Geometry check sheet. Reference: drawing and pictorial views, mm from the part's lowest x, y, z. Coordinates: 2 decimals unless noted, no trailing zeros. Write each loop counter-clockwise with the first axis right and the second up, starting at its lowest first coordinate (ties: lowest second). Pieces come first, ordered by that corner, then holes. Notation, with made-up numbers: M -4.75,17 L 22.25,17 A33 cw 22.25,45 Z; hole C 26,36.25 d4. An arc over 180 degrees is marked long. One line per item, written item: value.
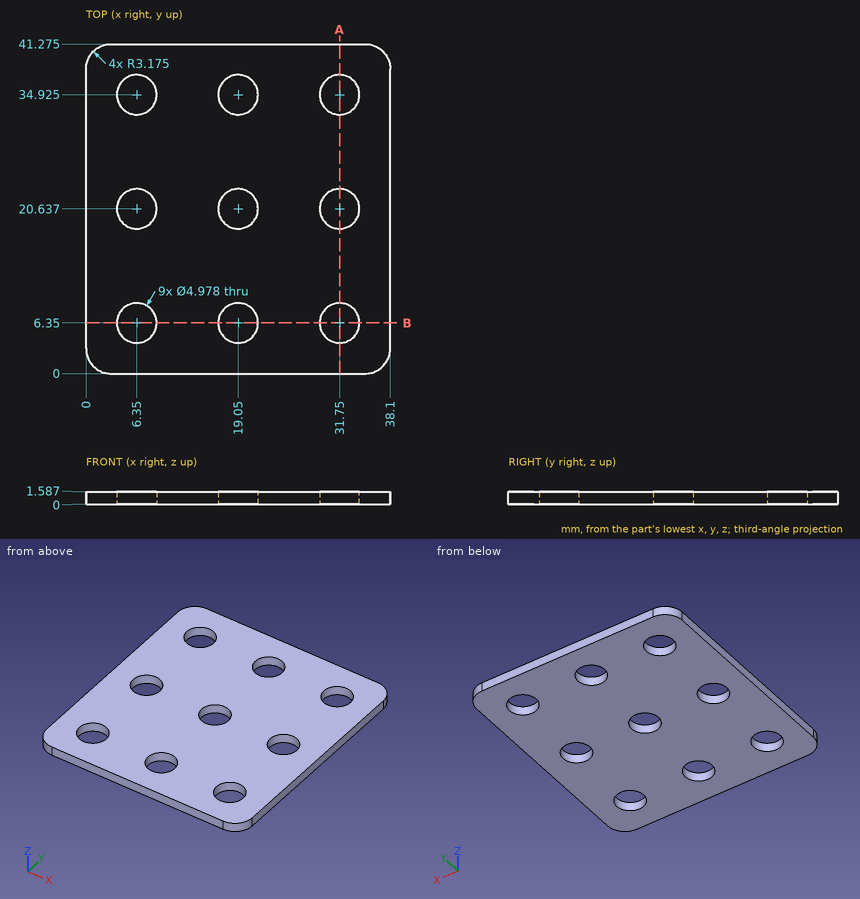
Item 1: Cross-section at A-A, the plane x = 31.75. Enter the section's corners in (y, z) (1 decimal).
The answers:
outline: M 0,0 L 3.9,0 L 3.9,1.6 L 0,1.6 Z; M 8.8,0 L 18.1,0 L 18.1,1.6 L 8.8,1.6 Z; M 23.1,0 L 32.4,0 L 32.4,1.6 L 23.1,1.6 Z; M 37.4,0 L 41.3,0 L 41.3,1.6 L 37.4,1.6 Z
Item 2: Go/stop test with flat-tipped pins: P1, Ø3, axis at x = 6.35, y = 34.925, coming from the +Z side; P2, Ø6.5, axis at x = 31.75, y = 6.35, coming from the -Z side. Record where each tip stops, or that it passes through.
The answers:
P1: passes through
P2: stops at z = 0
Item 3: Cross-section at B-B, the plane y = 6.35. Enter the section's corners in (x, z).
The answers:
outline: M 0,0 L 3.86,0 L 3.86,1.59 L 0,1.59 Z; M 8.84,0 L 16.56,0 L 16.56,1.59 L 8.84,1.59 Z; M 21.54,0 L 29.26,0 L 29.26,1.59 L 21.54,1.59 Z; M 34.24,0 L 38.1,0 L 38.1,1.59 L 34.24,1.59 Z
Item 4: Scan lines: line 1 (Y direction, x = 6.35, z = 0.8) (1 decimal); line 2 (X direction, y = 6.5, z = 1.3) (1 decimal); line 3 (Y direction, x = 34, z = 0.7) (1 decimal). Record each from-to range of solid material in increasing order.
The answers:
line 1: y = 0 to 3.9, 8.8 to 18.1, 23.1 to 32.4, 37.4 to 41.3
line 2: x = 0 to 3.9, 8.8 to 16.6, 21.5 to 29.3, 34.2 to 38.1
line 3: y = 0 to 5.3, 7.4 to 19.6, 21.7 to 33.9, 36 to 41.3
